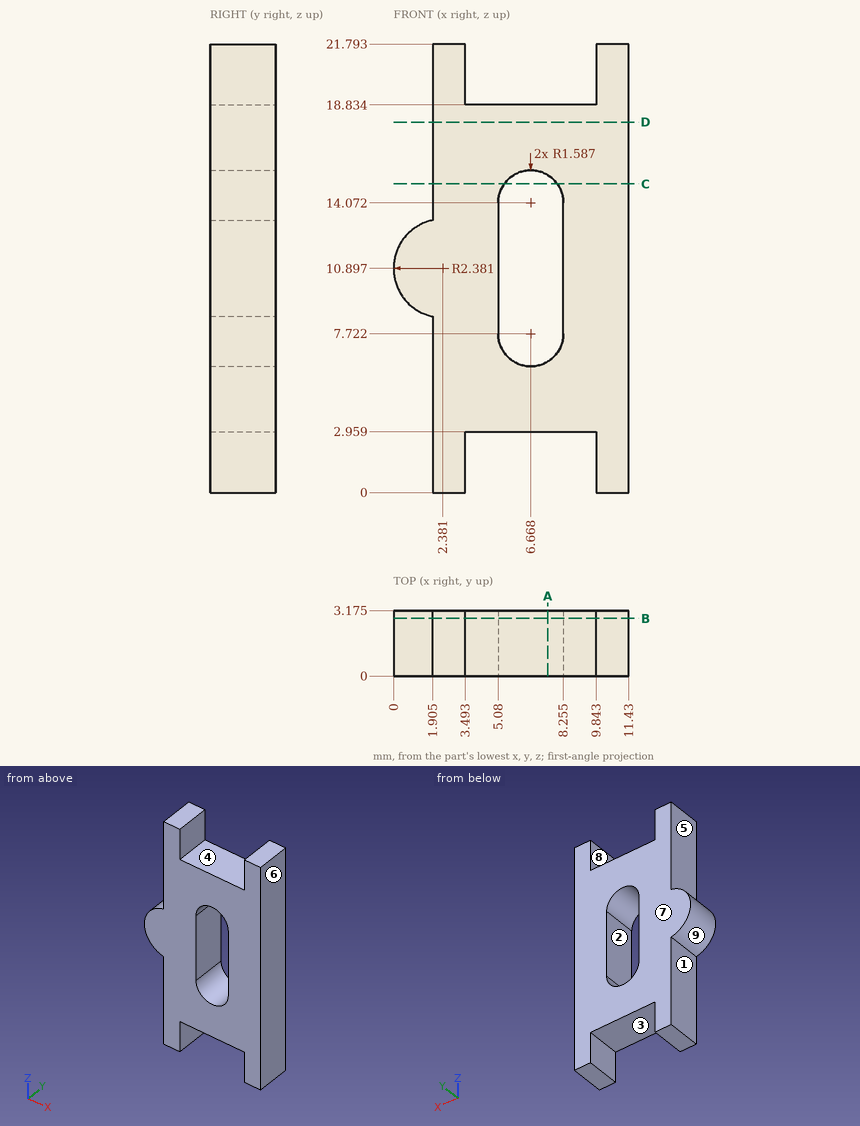
For this review, use the dimensioned drawing (mm, ordinates from the lowest corner) and the shaded views. A direction names the side the tool comes from. Give positions to 0.01 mm unless a question says otherwise; leave off trailing zeros. Order: outer loops, then holes, each group sorted by start corner. A loop starts at its lowest first (then second) coordinate and runs counter-clockwise, first axis right, second up.
1) The part is to be moulded in two halves that separate along X. For the marked faces 6, 7, 8 and 9, say which applies: released by +X, released by -X, zero draft, split by the parting line, or undercut.
2) Take a section at A-A (x = 7.5). Give the boundary of the cut face in (y, z) (1 decimal).
3) Wall thickness on line 1 (X direction, y = 0.75, z = 1.25) (1 decimal); line 2 (X direction, y = 2.65, z = 3.5) (1 decimal); line 3 (Z direction, x = 7, y = 2.5) (1 decimal): over which ranges is each line inside the solid? List them lowest first.
4) Insertion check: pin 1 (0.9 mm diameter, centred on y = 1.5, z = 20, fed in from -X) (1 decimal); pin 2 (1.5 mm diameter, centred on x = 6.5, y = 0.5, fed in from -Z). Each pin has a flat end and moves straight along its axis. Give the tip position at first contact, or say it passes through.
5) Take a section at D-D (z = 18). Give the boundary of the cut face in (x, y) (1 decimal).
6) Take a section at B-B (y = 2.8). Give the boundary of the cut face in (x, z) (1 decimal).
7) For the marked faces 1, 2, 3, 4 and 5, list the 3-axis set-ups (+Z, -Z, +X, -X, +Y, -Y) from which the entire face can be reached by the end or side of a thin tool; tool diameter is ignored.
8) Take a section at C-C (z = 15). Give the boundary of the cut face in (x, y) (1 decimal).
Derived:
1. face 6: released by +X
1. face 7: zero draft
1. face 8: undercut
1. face 9: released by -X
2. outline: (0, 3) - (3.2, 3) - (3.2, 6.4) - (0, 6.4) - close; (0, 15.4) - (3.2, 15.4) - (3.2, 18.8) - (0, 18.8) - close
3. line 1: x = 1.9 to 3.5, 9.8 to 11.4
3. line 2: x = 1.9 to 11.4
3. line 3: z = 3 to 6.2, 15.6 to 18.8
4. pin 1: stops at x = 1.9
4. pin 2: stops at z = 2.96
5. outline: (1.9, 0) - (11.4, 0) - (11.4, 3.2) - (1.9, 3.2) - close
6. outline: (1.9, 0) - (3.5, 0) - (3.5, 3) - (9.8, 3) - (9.8, 0) - (11.4, 0) - (11.4, 21.8) - (9.8, 21.8) - (9.8, 18.8) - (3.5, 18.8) - (3.5, 21.8) - (1.9, 21.8) - (1.9, 13.2) arc R2.4 ccw to (1.9, 8.6) - close; hole (5.1, 7.7) arc R1.6 ccw to (8.3, 7.7) - (8.3, 14.1) arc R1.6 ccw to (5.1, 14.1) - close
7. face 1: -Z, -X, +Y, -Y
7. face 2: +Y, -Y
7. face 3: -Z, +Y, -Y
7. face 4: +Z, +Y, -Y
7. face 5: +Z, -X, +Y, -Y
8. outline: (1.9, 0) - (5.4, 0) - (5.4, 3.2) - (1.9, 3.2) - close; (8, 0) - (11.4, 0) - (11.4, 3.2) - (8, 3.2) - close
